```python
from build123d import *

# Parameters (mm, degrees)
BOSS_EXTRUDE1_DEPTH = 10
FILLET3_R           = 0.1


with BuildPart() as part:
    # airflap → Boss-Extrude1 (new body)
    with BuildSketch(Plane(origin=(0, 0, 0), x_dir=(0, 0, -1), z_dir=(1, 0, 0))):
        with BuildLine():
            Line((3.897114317, 2.25), (4.330127019, 2.5))
            ThreePointArc((4.330127019, 2.5), (5, 0), (4.330127019, -2.5))
            Line((4.330127019, -2.5), (3.897114317, -2.25))
            ThreePointArc((3.897114317, -2.25), (4.5, 0), (3.897114317, 2.25))
        make_face()
    extrude(amount=BOSS_EXTRUDE1_DEPTH)

    # Fillet3
    fillet3_edges = [part.edges().sort_by_distance(p)[0] for p in [
        (10, 0, -5),
        (5, 2.5, -4.330127019),
        (5, -2.5, -4.330127019),
    ]]
    fillet(fillet3_edges, radius=FILLET3_R)


solid = part.part
```
Can you work these out from the model? Positions are in its coordinate system, mm. Round coordinates to 2 decimals unless told otherwise and drop trailing zeros. Order: outer loops, then holes, each group sorted by start corner. A loop starts at its lowest first (then second) coordinate and runs counter-clockwise, first axis right, second up. Notation, with made-up numbers: (-14, 34) -> (43, 34) arc R11 cw to (43, 50) -> close; hole circle Ø7 at (12, 63). An arc over 180 degrees is marked (long way). Return JSON: item names as keys, results as strings. Group by question number.
1. We'd pull the mould along Y, two halves only. Please class faces 1 (the face through (4.9, 0, -4.5)), 2 (the face through (0, 0, -4.7)), 3 (the face through (5, 0, -5)): released by +Y, released by -Y, zero draft, split by the parting line, or undercut.
2. If we section it at A-A, the plane z = -4.15: Write out the boundary of the cut face in (x, y).
3. If we section it at B-B, the plane x = 1.5: Write out the boundary of the cut face in (y, z), then the cut area to 3 significant figures.
4. I need wall thicknesses on line 1 (Y direction, x = 9, z = -4); line 2 (Z direction, x = 1.25, y = 0); line 3 (Z direction, x = 4.25, y = 0.95). Which ranges of each line are inside material? Lowest first, please. Write a range as [from, to].
Output values:
{
 "1": {"face 1": "undercut", "face 2": "zero draft", "face 3": "split by the parting line"},
 "2": {"outline": "(0, -2.4) -> (10, -2.4) -> (10, -1.74) -> (0, -1.74) -> close; (0, 1.74) -> (10, 1.74) -> (10, 2.4) -> (0, 2.4) -> close"},
 "3": {"outline": "(-2.45, -4.24) arc R0.1 ccw to (-2.41, -4.38) arc R5 ccw to (2.41, -4.38) arc R0.1 ccw to (2.45, -4.24) -> (2.25, -3.9) arc R4.5 cw to (-2.25, -3.9) -> close", "area": "2.48 mm²"},
 "4": {"line 1": "[-2.31, -2.06], [2.06, 2.31]", "line 2": "[-5, -4.5]", "line 3": "[-4.91, -4.4]"}
}
